Autodesk Inventor part; units mm, degrees
ref_plane "XZ Plane" through (0, 0, 0) normal (0, 1, 0) x (-1, 0, 0)
ref_plane "XY Plane" through (0, 0, 0) normal (0, 0, 1) x (1, 0, 0)
sketch "Sketch1" plane through (0, 0, 0) normal (1, 0, 0) x (0, 1, 0)
  line L0 (5.5, 0) -> (5.5, -14)
  line L1 (3, -18.3301) -> (3, -54.5301)
  line L2 (5.5, -14) -> (3, -18.3301)
  line L3 (6.4, -14.2412) -> (6.4, 0)
  line L4 (3.9, -54.5301) -> (3.9, -18.5713)
  line L5 (3.9, -18.5713) -> (6.4, -14.2412)
  line L6 (5.5, 0) -> (6.4, 0)
  line L7 (3, -54.5301) -> (3.9, -54.5301)
  line L8 (0, 0) -> (0, -13.4329) construction
  dimension "d7" = 5.5
  dimension "d8" = 3
  dimension "d9" = 150
  dimension "d10" = 0.9
  dimension "d11" = 0.9
  dimension "d12" = 0.9
  dimension "d13" = 14
  dimension "d14" = 36.2
revolve "Revolution1" add sketch "Sketch1" angle 360 about axis through (0, 0, 0) along (0, 0, -1)
ref_plane "Work Plane2" through (7, 0, 0) normal (1, 0, 0) x (0, 1, 0)
sketch "Sketch2" plane through (7, 0, 0) normal (1, 0, 0) x (0, 1, 0)
  line L0 (0, 0) -> (0, -5) construction
  line L1 (0, -5) -> (3.4, -5) construction
  circle A0 centre (3.4, -5) radius 1
  dimension "d18" = 5
  dimension "d19" = 3.4
  dimension "d20" = 2
extrude "Extrusion1" cut sketch "Sketch2" against normal blind 5
pattern_circular "Circular Pattern1" count 4 over 360 about axis through (0, 0, -7) along (0, 0, -1) of "Extrusion1"
properties part number "oxidizer"
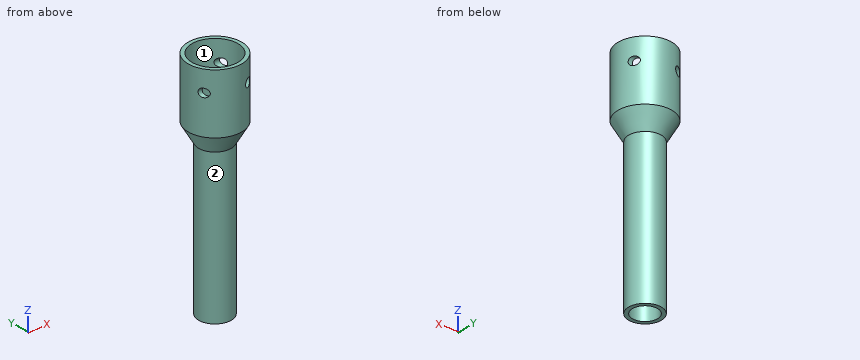
Here's how the part is built. I have some questions about the finished solid (model axes, mm). Face numbers are marked on the shaded views. Give positions to 0.01 mm unless a question says otherwise; leave off trailing zeros. Order: outer loops, then holes, each group sorted by start corner. A loop starts at its lowest first (then second) coordinate and runs counter-clockwise, first axis right, second up. Notation, with made-up numbers: (47, 7) -> (91, 7) arc R26 ccw to (91, 32) -> close; hole circle Ø6 at (-28.75, -16.75). An arc over 180 degrees is marked (long way). Use CSV: the item, a comma, the result in double quotes. Start each with the question number.
Item 1: Suppose I cut it at C-C (z = -41). List the corners of the cut face in (x, y) for me, and give its area (3 significant figures).
Item 2: Suppose I cut it at A-A (y = 0). List the corners of the cut face in (x, z) for me, and give its area (3 significant figures).
Item 3: Suppose I cut it at B-B (z = -5). List the corners of the cut face in (x, y) for me, and give its area (3 significant figures).
Item 4: I'm going to push flat-ended pins straight in: P1, Ø2, axis at y = 1.5, z = -8.5, coming from the -X side; P2, Ø3, axis at x = -3.5, z = -41.5, coming from the -Y side; P3, Ø3, axis at x = -3.4, z = -5, coming from the +Y side. Where does each tip first touch, or does it pass through?
Item 5: Suppose I cut it at D-D (z = -17.5). List the corners of the cut face in (x, y) for me.
Item 6: Thinking about a two-plate mould opening in X: for the marked faces 1 and 2, which applies, pulls with the +X half, pulls with the -X half, needs draft (parallel to the pull), parting line crosses it, or undercut?
Item 7: If I drill on probe 1 along X at (y, z) = (-0.25, -38); probe 2 along X at (y, z) = (0, -10.5); probe 3 along Y at (x, z) = (-2, -18.5), over which ranges is the centre line in solid material (lowest first)? Write a range as [from, to].
Answer block:
1,outline,"circle Ø7.8 at (0, 0); hole circle Ø6 at (0, 0)"
1,area,"19.5 mm^2"
2,outline,"(-6.4, -14.24) -> (-3.9, -18.57) -> (-3.9, -54.53) -> (-3, -54.53) -> (-3, -18.33) -> (-5.5, -14) -> (-5.5, 0) -> (-6.4, 0) -> close; (3, -54.53) -> (3.9, -54.53) -> (3.9, -18.57) -> (6.4, -14.24) -> (6.4, 0) -> (5.5, 0) -> (5.5, -14) -> (3, -18.33) -> close"
2,area,"99.4 mm^2"
3,outline,"(-5.93, -2.4) -> (-4.95, -2.4) arc R5.5 cw to (-4.4, 3.3) -> (-4.4, 4.65) arc R6.4 ccw to start; (-4.65, -4.4) arc R6.4 ccw to (2.4, -5.93) -> (2.4, -4.95) arc R5.5 cw to (-3.3, -4.4) -> close; (-2.4, 4.95) arc R5.5 cw to (3.3, 4.4) -> (4.65, 4.4) arc R6.4 ccw to (-2.4, 5.93) -> close; (4.4, -4.65) arc R6.4 ccw to (5.93, 2.4) -> (4.95, 2.4) arc R5.5 cw to (4.4, -3.3) -> close"
3,area,"24.7 mm^2"
4,P1,"stops at x = -6.38"
4,P2,"stops at y = -3.35"
4,P3,"stops at y = 6.11"
5,outline,"circle Ø9.04 at (0, 0); hole circle Ø6.96 at (0, 0)"
6,face 1,"undercut"
6,face 2,"parting line crosses it"
7,probe 1,"x = [-3.89, -2.99], [2.99, 3.89]"
7,probe 2,"x = [-6.4, -5.5], [5.5, 6.4]"
7,probe 3,"y = [-3.4, -2.24], [2.24, 3.4]"
